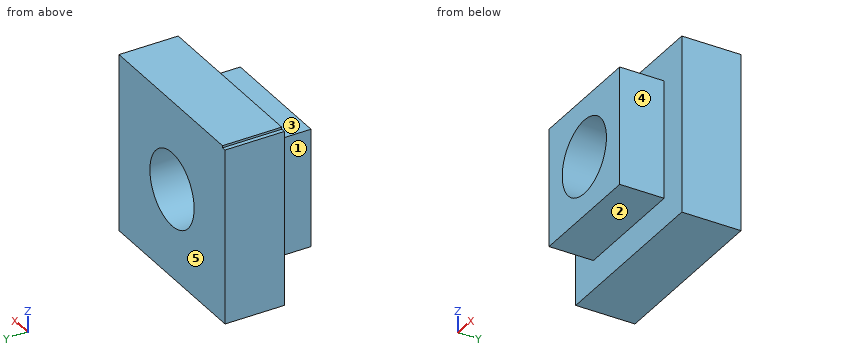
from build123d import *

# Parameters (mm, degrees)
F0_W     = 101.6
F0_H     = 101.6
F0_R     = 31.75
F1_DEPTH = 38.1
F2_R     = 31.75
F3_DEPTH = 50.8


with BuildPart() as f1:
    # F0 (on Front) → F1 (new body)
    with BuildSketch(Plane.XZ):
        Rectangle(F0_W, F0_H)
        Circle(F0_R, mode=Mode.SUBTRACT)
    extrude(amount=F1_DEPTH)

    # F2 (on Front) → F3 (join)
    with BuildSketch(Plane.XZ):
        Polygon((-72.544911, 76.2), (-72.544911, 74.35935), (-76.2, 74.35935), (-76.2, -76.2), (76.2, -76.2), (76.2, 76.2), align=None)
        Circle(F2_R, mode=Mode.SUBTRACT)
    extrude(amount=-F3_DEPTH)


solid = f1.part
Model file for the job. Use its own axes, mm. Face numbers are marked on the shaded views. A direction names the side the tool comes from. Give positions to 0.01 mm unless a question says otherwise; leave off trailing zeros. Order: outer loops, then holes, each group sorted by start corner. A loop starts at its lowest first (then second) coordinate and runs counter-clockwise, first axis right, second up. Notation, with made-up numbers: M -39,17.5 L -24,17.5 A21 cw -24,24.5 Z; hole C 33.5,-10.75 d8. An arc over 180 degrees is marked long. Put each result on its own line as item: value. Start each with the question number.
(1) Drill centre lines: L1, parallel to Z at x = 0, y = -15.5; L2, parallel to Z at x = 0, y = 16; L3, parallel to Y at x = -26, z = -67.5. Where is each one in solid material? Low to high. Write a range as [from, to].
(2) Band-saw the part on C-C on y = 15. Give the cut face in (x, z), then the cut area to 3 significant figures.
(3) Band-saw the part on A-A on z = 0. Give the cut face in (x, y), then the cut area to 3 significant figures.
(4) Pin check, flat tips, straight feed: pin 1 Ø0.6 at (y, z) = (13.5, 75.5) entering from -X; pin 2 Ø8 at (y, z) = (-1.5, -44.5) entering from -X; pin 3 Ø10 at (x, z) = (60.5, 15) entering from -Y; pin 4 Ø19 at (x, y) = (0.5, -27.5) entering from +Z. Stop position of each tip, or through.
(5) Tool access for the marked faces 1, 2, 3, 4 and 5: list every direction of +Z, -Z, +X, -X, +Y, -Y with a clear straight run to the whole face (end or side of a thin tool).
(6) Band-saw the part on B-B on x = 0. Give the cut face in (y, z).
(7) Band-saw the part on D-D on z = 35.5. Give the cut face in (x, y).
Results below:
1. L1: z = [-50.8, -31.75], [31.75, 50.8]
1. L2: z = [-76.2, -31.75], [31.75, 76.2]
1. L3: y = [0, 50.8]
2. outline: M -76.2,-76.2 L 76.2,-76.2 L 76.2,76.2 L -72.54,76.2 L -72.54,74.36 L -76.2,74.36 Z; hole C 0,0 d63.5
2. area: 20,100 mm2
3. outline: M -76.2,0 L -50.8,0 L -50.8,-38.1 L -31.75,-38.1 L -31.75,50.8 L -76.2,50.8 Z; M 31.75,-38.1 L 50.8,-38.1 L 50.8,0 L 76.2,0 L 76.2,50.8 L 31.75,50.8 Z
3. area: 5,970 mm2
4. pin 1: stops at x = -72.54
4. pin 2: stops at x = -76.2
4. pin 3: stops at y = 0
4. pin 4: stops at z = 50.8
5. face 1: +Z, -Z, -X, -Y
5. face 2: -Z, +X, -X, -Y
5. face 3: +Z, +X, -X, -Y
5. face 4: +Z, -Z, +X, -Y
5. face 5: +Z, -Z, +X, -X, +Y
6. outline: M -38.1,-50.8 L 0,-50.8 L 0,-76.2 L 50.8,-76.2 L 50.8,-31.75 L -38.1,-31.75 Z; M -38.1,31.75 L 50.8,31.75 L 50.8,76.2 L 0,76.2 L 0,50.8 L -38.1,50.8 Z
7. outline: M -76.2,0 L -50.8,0 L -50.8,-38.1 L 50.8,-38.1 L 50.8,0 L 76.2,0 L 76.2,50.8 L -76.2,50.8 Z
